Here's how the part is built. I have some questions about the finished solid (model axes, mm). A direction names the side the tool comes from. Give positions to 0.01 mm unless a question says otherwise; leave off trailing zeros. Loops run counter-clockwise (first coordinate to the right, second up) from the corner with the lowest first, then second, coordinate; pieces in that order, holes last. Notation, with made-up numbers: (-26.75, -36) - (12.25, -36) arc R28 ccw to (12.25, -11) - close; hole circle Ø9 at (80, -25.5). An arc over 180 degrees is marked (long way). Use a Markdown table: item, result.
from build123d import *

# Parameters (mm, degrees)
SKETCH_1_W          = 55
SKETCH_1_H          = 86
EXTRUDE_1_DEPTH     = 2
SKETCH_2_R          = 6.5
CUT_EXTRUDE_1_DEPTH = 52.198144498
SKETCH_3_R          = 1.6
CUT_EXTRUDE_2_DEPTH = 52.198144498
SKETCH_4_R          = 1.6
CUT_EXTRUDE_3_DEPTH = 52.198144498
SKETCH_7_R          = 17.5
CUT_EXTRUDE_6_DEPTH = 52.198144498
FILLET_2_R          = 5


with BuildPart() as part:
    # ｽｹｯﾁ1 → ﾎﾞｽ - 押し出し1 (new, symmetric)
    with BuildSketch(Plane.XY):
        Rectangle(SKETCH_1_W, SKETCH_1_H)
    extrude(amount=EXTRUDE_1_DEPTH, both=True)

    # ｽｹｯﾁ2 → ｶｯﾄ - 押し出し1 (cut, through all)
    with BuildSketch(Plane.XY.offset(2)):
        with Locations((7.5, 0)):
            Circle(SKETCH_2_R)
    extrude(amount=-CUT_EXTRUDE_1_DEPTH, mode=Mode.SUBTRACT)

    # ｽｹｯﾁ3 → ｶｯﾄ - 押し出し2 (cut, through all)
    with BuildSketch(Plane.XY.offset(2)):
        with Locations((-22.5, 38)):
            Circle(SKETCH_3_R)
        with Locations(Location((22.5, 38, 0), (0, 0, 180))):
            Circle(SKETCH_3_R)
        with Locations((22.5, -38)):
            Circle(SKETCH_3_R)
        with Locations(Location((-22.5, -38, 0), (0, 0, 180))):
            Circle(SKETCH_3_R)
    extrude(amount=-CUT_EXTRUDE_2_DEPTH, mode=Mode.SUBTRACT)

    # ｽｹｯﾁ4 → ｶｯﾄ - 押し出し3 (cut, through all)
    with BuildSketch(Plane(origin=(0, 0, -2), x_dir=(-1, 0, 0), z_dir=(0, 0, -1))):
        with Locations((-7.5, 16.215)):
            Circle(SKETCH_4_R)
        with Locations((-7.5, -16.215)):
            Circle(SKETCH_4_R)
    extrude(amount=-CUT_EXTRUDE_3_DEPTH, mode=Mode.SUBTRACT)

    # ｽｹｯﾁ7 → ｶｯﾄ - 押し出し6 (cut, through all)
    with BuildSketch(Plane.XY.offset(2)):
        with Locations((0, 43)):
            Circle(SKETCH_7_R)
        with Locations((0, -43)):
            Circle(SKETCH_7_R)
    extrude(amount=-CUT_EXTRUDE_6_DEPTH, mode=Mode.SUBTRACT)

    # ﾌｨﾚｯﾄ2
    fillet_2_edges = [part.edges().sort_by_distance(p)[0] for p in [
        (17.5, 43, 0),
        (-17.5, 43, 0),
        (-17.5, -43, 0),
        (17.5, -43, 0),
        (27.5, -43, 0),
        (-27.5, -43, 0),
        (-27.5, 43, 0),
        (27.5, 43, 0),
    ]]
    fillet(fillet_2_edges, radius=FILLET_2_R)


solid = part.part
(1) If I drill on line 1 (Y direction, x = -22.5, z = -0.35); line 2 (Y direction, x = 7.5, z = 0.15) (3 decimals); line 3 (Y direction, x = -23, z = 0.9), over which ranges is the centre line in solid material (lowest first)?
A:
| item | result |
|---|---|
| line 1 | -43 to -39.6, -36.4 to 36.4, 39.6 to 43 |
| line 2 | -27.189 to -17.815, -14.615 to -6.5, 6.5 to 14.615, 17.815 to 27.189 |
| line 3 | -42.97 to -39.52, -36.48 to 36.48, 39.52 to 42.97 |
(2) Suppose I cut it at B-B on x = 11.5. Write out the boundary of the cut face in (y, z), plus the area to 3 significant figures.
A:
| item | result |
|---|---|
| outline | (-29.81, -2) - (-5.12, -2) - (-5.12, 2) - (-29.81, 2) - close; (5.12, -2) - (29.81, -2) - (29.81, 2) - (5.12, 2) - close |
| area | 197 mm2 |
(3) Suppose I cut it at A-A on y = 0. Write out the boundary of the cut face in (x, z), plus the area to 3 significant figures.
A:
| item | result |
|---|---|
| outline | (-27.5, -2) - (1, -2) - (1, 2) - (-27.5, 2) - close; (14, -2) - (27.5, -2) - (27.5, 2) - (14, 2) - close |
| area | 168 mm2 |
(4) We'd pull the mould along Y, two halves only. Please class faces 4 (the face through (13.7, 1.95, 0.03)), 5 (the face through (21.76, 39.42, 0.03)), 6 (the face through (-26.07, -41.5, 0.03)), 7 (the face through (0, 1, 2)): pulls with the +Y half, pulls with the -Y half, needs draft (parallel to the pull), parting line crosses it, or undercut.
A:
| item | result |
|---|---|
| face 4 | undercut |
| face 5 | undercut |
| face 6 | pulls with the -Y half |
| face 7 | needs draft |
(5) Suppose I cut it at C-C on z = -1.2. Write out the boundary of the cut face in (x, y) (3 decimals), plus the area to 3 significant figures.
A:
| item | result |
|---|---|
| outline | (-27.5, -38) arc R5 ccw to (-22.5, -43) - (-21.937, -43) arc R5 ccw to (-17.062, -39.111) arc R17.5 cw to (17.062, -39.111) arc R5 ccw to (21.937, -43) - (22.5, -43) arc R5 ccw to (27.5, -38) - (27.5, 38) arc R5 ccw to (22.5, 43) - (21.937, 43) arc R5 ccw to (17.062, 39.111) arc R17.5 cw to (-17.062, 39.111) arc R5 ccw to (-21.937, 43) - (-22.5, 43) arc R5 ccw to (-27.5, 38) - close; hole circle Ø3.2 at (-22.5, -38); hole circle Ø3.2 at (-22.5, 38); hole circle Ø13 at (7.5, 0); hole circle Ø3.2 at (7.5, -16.215); hole circle Ø3.2 at (7.5, 16.215); hole circle Ø3.2 at (22.5, -38); hole circle Ø3.2 at (22.5, 38) |
| area | 3,550 mm2 |
(6) Will these pins go through, and if not, where does the flat tip stop? pin 1 (1.5 mm diameter, centred on x = -20.5, z = -0.5, fed in from +Y); pin 2 (2 mm diameter, centred on x = -10.5, z = 1.5, fed in from +Y); pin 3 (1 mm diameter, centred on x = 15, z = -1, fed in from -Y).
A:
| item | result |
|---|---|
| pin 1 | y = 42.95 |
| pin 2 | y = 29.81 |
| pin 3 | y = -34.88 |
(7) Suppose I cut it at D-D on x = -10.5. Write out the boundary of the cut face in (y, z), plus the area to 3 significant figures.
A:
| item | result |
|---|---|
| outline | (-29, -2) - (29, -2) - (29, 2) - (-29, 2) - close |
| area | 232 mm2 |
(8) On a 3-axis mill with a long thin cutter (end or side, diameter ignored), from which of +Z, -Z, +X, -X, +Y, -Y can I reach the whole of each face in a straight line? I mean faces 1 (the face through (18.783, -41.879, -0.028)), 2 (the face through (7.71, -14.63, -0.03)), 3 (the face through (-18.86, 41.94, 0.03)). Say none if no direction works.
A:
| item | result |
|---|---|
| face 1 | +Z, -Z, -Y |
| face 2 | +Z, -Z |
| face 3 | +Z, -Z, +Y |
